```python
from build123d import *

# Parameters (mm, degrees)
SKETCH1_R           = 10
BOSS_EXTRUDE1_DEPTH = 10
SKETCH2_W           = 20
SKETCH2_H           = 18
BOSS_EXTRUDE2_DEPTH = 2
SKETCH3_R           = 1
BOSS_EXTRUDE3_DEPTH = 2
SKETCH5_R           = 1.5
CUT_EXTRUDE1_DEPTH  = 2


with BuildPart() as part:
    # Sketch1 → Boss-Extrude1 (new body)
    with BuildSketch(Plane.XY):
        Circle(SKETCH1_R)
    extrude(amount=BOSS_EXTRUDE1_DEPTH)

    # Sketch2 → Boss-Extrude2 (add)
    with BuildSketch(Plane.XY.offset(10)):
        with Locations((0, -9)):
            Rectangle(SKETCH2_W, SKETCH2_H)
    extrude(amount=-BOSS_EXTRUDE2_DEPTH)

    # Sketch3 → Boss-Extrude3 (add)
    with BuildSketch(Plane(origin=(0, 0, 0), x_dir=(-1, 0, 0), z_dir=(0, 0, -1))):
        with Locations(Location((0, 0, 0), (0, 0, 180))):
            Circle(SKETCH3_R)
    extrude(amount=BOSS_EXTRUDE3_DEPTH)

    # Sketch5 → Cut-Extrude1 (cut)
    with BuildSketch(Plane(origin=(0, 0, 8), x_dir=(-1, 0, 0), z_dir=(0, 0, -1))):
        with Locations((-5.5, -14.5)):
            Circle(SKETCH5_R)
        with Locations((5.5, -14.5)):
            Circle(SKETCH5_R)
    extrude(amount=-CUT_EXTRUDE1_DEPTH, mode=Mode.SUBTRACT)


solid = part.part
```
Check sheet for the modelled part. Datum: model origin and axes. Units: mm. A direction names the side the tool comes from. Coordinates: 2 decimals unless noted, no trailing zeros. Loops run counter-clockwise (first coordinate to the right, second up) from the corner with the lowest first, then second, coordinate; pieces in that order, holes last. Notation, with made-up numbers: M -30.5,-12 L -16.5,-12 A13 cw -16.5,-3 Z; hole C 4,14.25 d6. An arc over 180 degrees is marked long. Answer as a JSON object with one key per item and string values.
1. Scan lines: L1, parallel to Z at x = 6, y = -5.5; L2, parallel to Z at x = 3, y = -13.25; L3, parallel to Y at x = 0.25, z = 1.25. Record each from-to range of solid material in increasing order. Write a range as from..to.
Outcome:
{"L1": "0..10", "L2": "8..10", "L3": "-10..10"}
2. Sectioned sample at C-C on x = 5.5. Record the cut outline in (y, z).
Outcome:
{"outline": "M -18,8 L -16,8 L -16,10 L -18,10 Z; M -13,8 L -8.35,8 L -8.35,0 L 8.35,0 L 8.35,10 L -13,10 Z"}
3. Depth check by flat-ended pin: P1, Ø3, axis at x = 4, z = 5, coming from the +Y side; P2, Ø2, axis at y = 6, z = 8.5, coming from the +X side; P3, Ø1.5, axis at x = 0, z = -1, coming from the +Y side. Enter the tip coordinate at first touch or a pass-through.
Outcome:
{"P1": "y = 9.68", "P2": "x = 8.66", "P3": "y = 1"}
4. Sectioned sample at A-A on y = -14.5. Record the cut outline in (x, z), and give its area (3 significant figures).
Outcome:
{"outline": "M -10,8 L -7,8 L -7,10 L -10,10 Z; M -4,8 L 4,8 L 4,10 L -4,10 Z; M 7,8 L 10,8 L 10,10 L 7,10 Z", "area": "28.0 mm²"}
5. Access from +Z, -Z, +X, -X, +Y, -Y to the whole of each face (thin tool, end or side, straight path). Record for faces 4 (the cylindrical face through (0, 1, -1)), 5 (the flat face through (10, -9, 9)).
Outcome:
{"face 4": "-Z", "face 5": "+Z, -Z, +X, +Y, -Y"}
6. Sectioned sample at B-B on x = 0. Record the cut outline in (y, z), and give its area (3 significant figures).
Outcome:
{"outline": "M -18,8 L -10,8 L -10,0 L -1,0 L -1,-2 L 1,-2 L 1,0 L 10,0 L 10,10 L -18,10 Z", "area": "220 mm²"}
7. Sectioned sample at D-D on z = 3.5. Record the cut outline in (x, y), and give its area (3 significant figures).
Outcome:
{"outline": "C 0,0 d20", "area": "314 mm²"}
8. Release check for a two-part mould opening along Y. For faces 1 (the flat face through (0, -13, 8)), 2 (the cylindrical face through (-1.302, 9.915, 4.93)), 3 (the cylindrical face through (6.7, -15.4, 9)) record: pulls with the +Y half, pulls with the -Y half, needs draft (parallel to the pull), parting line crosses it, or undercut.
Outcome:
{"face 1": "needs draft", "face 2": "parting line crosses it", "face 3": "undercut"}
